Verification items for this drawing (mm, ordinates from the low corner). Give positions to 0.01 mm unless a question says otherwise; leave off trailing zeros. Loops run counter-clockwise (first coordinate to the right, second up) from the corner with the lowest first, then second, coordinate; pieces in that order, holes last. Notation, with made-up numbers: (37.5, -11.75) - (82.5, -11.75) arc R18 cw to (82.5, 17.25) - close; hole circle Ø5 at (1, 40.25). An arc over 180 degrees is marked (long way). Write item = value, one per line. Start each with the question number.
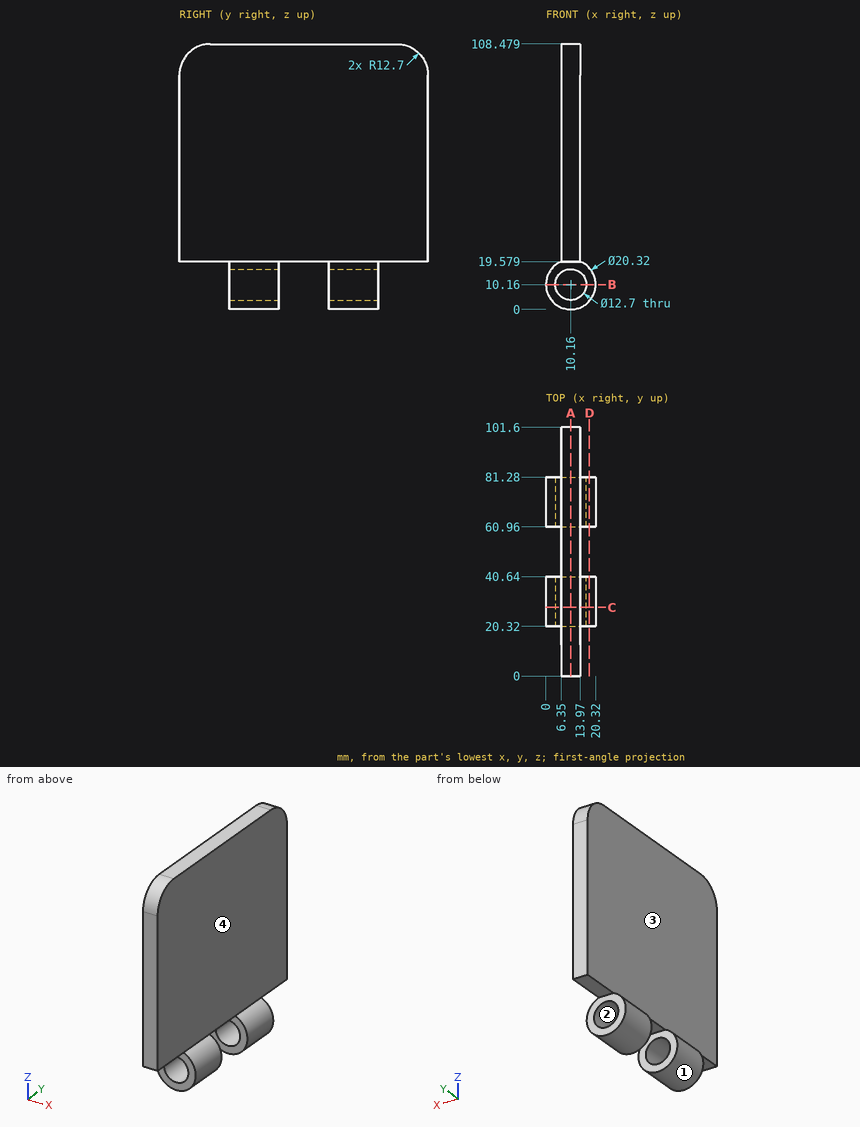
1) Cross-section at D-D on x = 17.75. Enter the section's corners in (y, z).
2) Cross-section at A-A on x = 10.16. Enter the section's corners in (y, z), and give its area (3 significant figures).
3) Cross-section at C-C on y = 28. Enter the section's corners in (x, z), and give its area (3 significant figures).
4) Material ranges on line 1 along Z through (x, y) = (10.75, 32); line 2 along Z through (x, y) = (9.25, 12.5); line 3 along X through (y, z) = (59, 82), recorded low to high.
5) Release check for a two-part mould opening along X. For the marked faces 1, 2, 3 and 4 record: pulls with the +X half, pulls with the -X half, needs draft (parallel to the pull), parting line crosses it, or undercut.
6) Cross-section at B-B on z = 10.16. Enter the section's corners in (x, y).
7) Gauge pin test, flat ends, axial feed: P1, Ø3, axis at y = 80, z = 70.5, coming from the +X side; P2, Ø4, axis at y = 51, z = 51.5, coming from the -X side; P3, Ø6, axis at x = 11.5, y = 95, coming from the -Z side. Record the tip position at first contact, or that the pin passes through.
Checked values:
q1.outline = (20.32, 3.41) - (40.64, 3.41) - (40.64, 16.91) - (20.32, 16.91) - close; (60.96, 3.41) - (81.28, 3.41) - (81.28, 16.91) - (60.96, 16.91) - close
q2.outline = (0, 19.58) - (20.32, 19.58) - (20.32, 16.51) - (40.64, 16.51) - (40.64, 19.58) - (60.96, 19.58) - (60.96, 16.51) - (81.28, 16.51) - (81.28, 19.58) - (101.6, 19.58) - (101.6, 95.78) arc R12.7 ccw to (88.9, 108.48) - (12.7, 108.48) arc R12.7 ccw to (0, 95.78) - close; (20.32, 0) - (40.64, 0) - (40.64, 3.81) - (20.32, 3.81) - close; (60.96, 0) - (81.28, 0) - (81.28, 3.81) - (60.96, 3.81) - close
q2.area = 9,240 mm²
q3.outline = (6.35, 19.58) arc R10.16 ccw (long way) to (13.97, 19.58) - (13.97, 108.48) - (6.35, 108.48) - close; hole circle Ø12.7 at (10.16, 10.16)
q3.area = 871 mm²
q4.line_1 = 0.02 to 3.84, 16.48 to 108.48
q4.line_2 = 19.58 to 108.48
q4.line_3 = 6.35 to 13.97
q5.face_1 = parting line crosses it
q5.face_2 = undercut
q5.face_3 = pulls with the -X half
q5.face_4 = pulls with the +X half
q6.outline = (0, 20.32) - (3.81, 20.32) - (3.81, 40.64) - (0, 40.64) - close; (0, 60.96) - (3.81, 60.96) - (3.81, 81.28) - (0, 81.28) - close; (16.51, 20.32) - (20.32, 20.32) - (20.32, 40.64) - (16.51, 40.64) - close; (16.51, 60.96) - (20.32, 60.96) - (20.32, 81.28) - (16.51, 81.28) - close
q7.P1 = 13.97
q7.P2 = 6.35
q7.P3 = 19.58
